Part print with two shaded views. Sizes in mm from the minimum x, y, z corner. A direction names the side the tool comes from. Give positions to 0.01 mm unless a question says otherwise; leave off trailing zeros. Order: outer loops, then holes, each group sorted by start corner. A loop starts at its lowest first (then second) coordinate and runs counter-clockwise, first axis right, second up. Notation, with made-up numbers: M -24,73.5 L -20,73.5 A21 cw -20,107.5 Z; hole C 66.5,-15.75 d5. An arc over 180 degrees is marked long. Return JSON: item names as keys, results as strings.
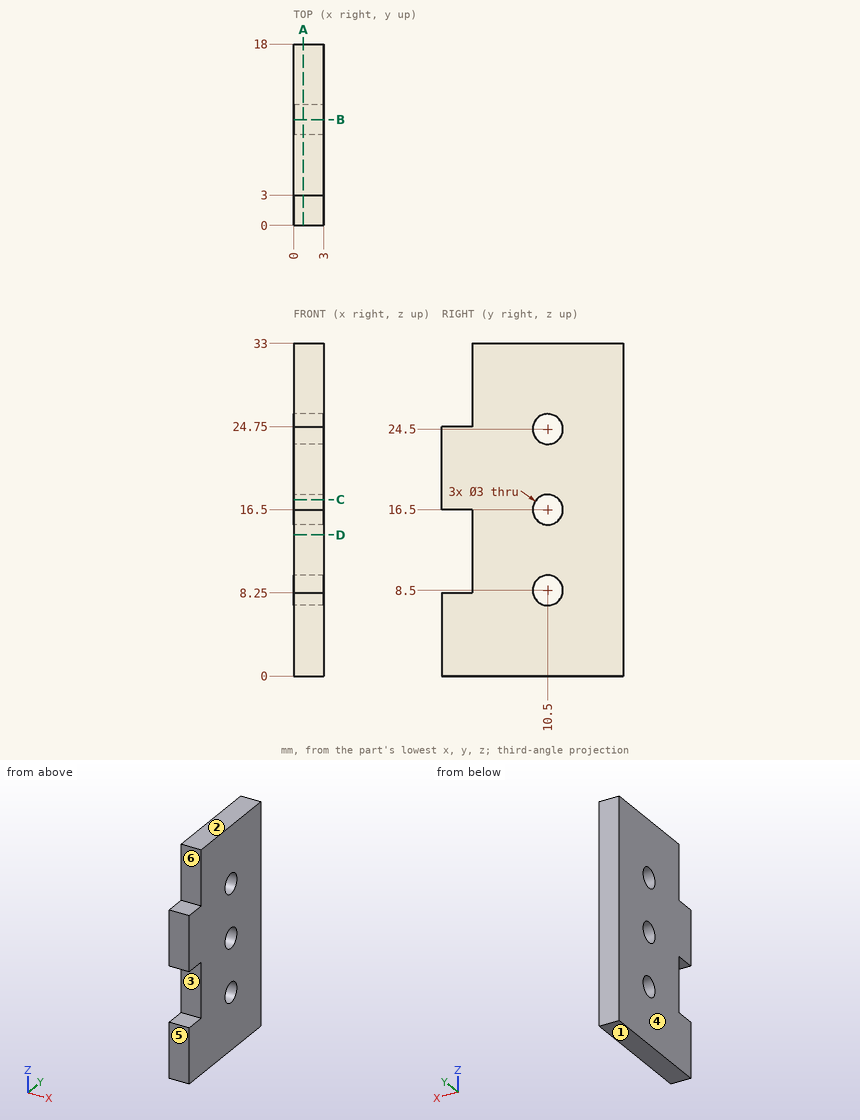
Q1. Band-saw the part on B-B (y = 10.5). Give the cut face in (x, z).
Established:
{"outline": "M 0,0 L 3,0 L 3,7 L 0,7 Z; M 0,10 L 3,10 L 3,15 L 0,15 Z; M 0,18 L 3,18 L 3,23 L 0,23 Z; M 0,26 L 3,26 L 3,33 L 0,33 Z"}
Q2. Band-saw the part on A-A (x = 0.95). Give the cut face in (y, z), then the cut area to 3 significant figures.
Established:
{"outline": "M 0,0 L 18,0 L 18,33 L 3,33 L 3,24.75 L 0,24.75 L 0,16.5 L 3,16.5 L 3,8.25 L 0,8.25 Z; hole C 10.5,8.5 d3; hole C 10.5,16.5 d3; hole C 10.5,24.5 d3", "area": "523 mm²"}
Q3. Probe line 1 along Z through (x, y) = (1.5, 10.5); line 2 along Z through (x, y) = (0.6, 1.75); line 3 along Y through (x, z) = (1.8, 31). List the from-to ranges inside material, lowest first.
Established:
{"line 1": "z = 0 to 7, 10 to 15, 18 to 23, 26 to 33", "line 2": "z = 0 to 8.25, 16.5 to 24.75", "line 3": "y = 3 to 18"}
Q4. 3-axis set-ups, long thin cutter, end or side, ignore diameter. For the marked faces 5 and 6: which of +Z, -Z, +X, -X, +Y, -Y reach the whole face in a straight line?
Established:
{"face 5": "+Z, -Z, +X, -X, -Y", "face 6": "+Z, +X, -X, -Y"}
Q5. Band-saw the part on C-C (z = 17.5). Give the cut face in (x, y).
Established:
{"outline": "M 0,0 L 3,0 L 3,9.38 L 0,9.38 Z; M 0,11.62 L 3,11.62 L 3,18 L 0,18 Z"}
Q6. Two-plate mould, pull along Z, no slides. Class the marked faces 1, 2, 3 and 4: +Z half, -Z half, draft (parallel to the pull), parting line (faces both ways), or undercut.
Established:
{"face 1": "-Z half", "face 2": "+Z half", "face 3": "undercut", "face 4": "draft"}
Q7. Pin check, flat tips, straight feed: pin 1 (0.9 mm diameter, centred on x = 2, y = 2, fed in from -Z); pin 2 (0.9 mm diameter, centred on x = 1.5, y = 1, fed in from +Z); pin 3 (2.5 mm diameter, centred on y = 10.5, z = 24.5, fed in from -X). Stop position of each tip, or through.
Established:
{"pin 1": "stops at z = 0", "pin 2": "stops at z = 24.75", "pin 3": "passes through"}
Q8. Band-saw the part on D-D (z = 14). Give the cut face in (x, y), then the cut area to 3 significant figures.
Established:
{"outline": "M 0,3 L 3,3 L 3,18 L 0,18 Z", "area": "45.0 mm²"}
